```python
from build123d import *

# Parameters (mm, degrees)
SKETCH_W        = 154
SKETCH_H        = 107
PAD_DEPTH       = 20
SKETCH001_W     = 151.5
SKETCH001_H     = 105
POCKET_DEPTH    = 5.5
SKETCH002_W     = 148
SKETCH002_H     = 101
POCKET001_DEPTH = 10.5
SKETCH003_R     = 5
POCKET002_DEPTH = 4.001
SKETCH004_R     = 2.5
PAD001_DEPTH    = 9
PAD001_TAPER    = -15


with BuildPart() as part:
    # Sketch → Pad (new body)
    with BuildSketch(Plane.XY):
        Rectangle(SKETCH_W, SKETCH_H)
    extrude(amount=PAD_DEPTH)

    # Sketch001 (on Face6 of Pad) → Pocket (cut)
    with BuildSketch(Plane.XY.offset(20)):
        Rectangle(SKETCH001_W, SKETCH001_H)
    extrude(amount=-POCKET_DEPTH, mode=Mode.SUBTRACT)

    # Sketch002 (on Face11 of Pocket) → Pocket001 (cut)
    with BuildSketch(Plane.XY.offset(14.5)):
        Rectangle(SKETCH002_W, SKETCH002_H)
    extrude(amount=-POCKET001_DEPTH, mode=Mode.SUBTRACT)

    # Sketch003 (on Face16 of Pocket001) → Pocket002 (cut, through all)
    with BuildSketch(Plane.XY.offset(4)):
        Circle(SKETCH003_R)
    extrude(amount=-POCKET002_DEPTH, mode=Mode.SUBTRACT)

    # Sketch004 (on Face12 of Pocket002) → Pad001 (join)
    with BuildSketch(Plane.XY.offset(4)):
        with Locations((-37, 25)):
            Circle(SKETCH004_R)
        with Locations((37, 25)):
            Circle(SKETCH004_R)
        with Locations((37, -25)):
            Circle(SKETCH004_R)
        with Locations((-37, -25)):
            Circle(SKETCH004_R)
    extrude(amount=PAD001_DEPTH, taper=PAD001_TAPER)


solid = part.part
```
CAD build for the part. Positions are in the model's coordinates, mm. A direction names the side the tool comes from. Round coordinates to 2 decimals unless told otherwise and drop trailing zeros. Loops run counter-clockwise (first coordinate to the right, second up) from the corner with the lowest first, then second, coordinate; pieces in that order, holes last. Notation, with made-up numbers: (-17.5, 0.25) - (37.5, 0.25) arc R14 ccw to (37.5, 26.25) - close; hole circle Ø8 at (46, 66). An arc over 180 degrees is marked (long way). Return JSON: item names as keys, results as strings. Group by question number.
Q1. Tool access for faces 1 (the face through (75.75, -1, 17)), 2 (the face through (-1, 13, 0)), 3 (the face through (40.295, -23.962, 7.563)): list every direction of +Z, -Z, +X, -X, +Y, -Y with a clear straight run to the whole face (end or side of a thin tool).
Q2. Band-saw the part on A-A on y = 0. Give the cut face in (x, z).
Q3. Band-saw the part on B-B on z = 7.25. Give the cut face in (x, y), plus the area to 3 significant figures.
Q4. Band-saw the part on C-C on x = -29. Give the cut face in (y, z), plus the area to 3 significant figures.
Q5. Flat gauge pins, fed straight in: pin 1 Ø5 at (x, y) = (-36.5, 27) entering from +Z; pin 2 Ø8 at (x, y) = (44.5, 18.5) entering from +Z. Where does each tip first touch, or does it go through?
Q6. Drill centre lines: line 1 along X through (y, z) = (38.5, 8.5); line 2 along Y through (x, z) = (-1.5, 15.75); line 3 along Y through (x, z) = (0, 2.8). Where is each one in solid material? Low to high. Write a range as [from, to].
Q7. Band-saw the part on D-D on y = -16.5. Give the cut face in (x, z), plus the area to 3 significant figures.
Q8. Two-plate mould, pull along Y, no slides. Class faces 4 (the face through (-77, -1, 10)), 5 (the face through (-1, 12, 4)), 6 (the face through (-1, -52.5, 17)), 7 (the face through (-1, 53.5, 10)): +Y half, -Y half, draft (parallel to the pull), parting line (faces both ways), or undercut.
Solutions:
{
 "1": {"face 1": "+Z", "face 2": "-Z, +X, -X, +Y, -Y", "face 3": "none"},
 "2": {"outline": "(-77, 0) - (-5, 0) - (-5, 4) - (-74, 4) - (-74, 14.5) - (-75.75, 14.5) - (-75.75, 20) - (-77, 20) - close; (5, 0) - (77, 0) - (77, 20) - (75.75, 20) - (75.75, 14.5) - (74, 14.5) - (74, 4) - (5, 4) - close"},
 "3": {"outline": "(-77, -53.5) - (77, -53.5) - (77, 53.5) - (-77, 53.5) - close; circle Ø6.74 at (-37, -25); circle Ø6.74 at (-37, 25); circle Ø6.74 at (37, -25); circle Ø6.74 at (37, 25); hole (-74, -50.5) - (74, -50.5) - (74, 50.5) - (-74, 50.5) - close", "area": "1,670 mm^2"},
 "4": {"outline": "(-53.5, 0) - (53.5, 0) - (53.5, 20) - (52.5, 20) - (52.5, 14.5) - (50.5, 14.5) - (50.5, 4) - (-50.5, 4) - (-50.5, 14.5) - (-52.5, 14.5) - (-52.5, 20) - (-53.5, 20) - close", "area": "502 mm^2"},
 "5": {"pin 1": "stops at z = 13", "pin 2": "stops at z = 4"},
 "6": {"line 1": "x = [-77, -74], [74, 77]", "line 2": "y = [-53.5, -52.5], [52.5, 53.5]", "line 3": "y = [-53.5, -5], [5, 53.5]"},
 "7": {"outline": "(-77, 0) - (77, 0) - (77, 20) - (75.75, 20) - (75.75, 14.5) - (74, 14.5) - (74, 4) - (-74, 4) - (-74, 14.5) - (-75.75, 14.5) - (-75.75, 20) - (-77, 20) - close", "area": "693 mm^2"},
 "8": {"face 4": "draft", "face 5": "undercut", "face 6": "undercut", "face 7": "+Y half"}
}
